```python
from build123d import *

# Parameters (mm, degrees)
SKETCH2_R           = 1
SKETCH2_R_2         = 7.975
BOSS_EXTRUDE1_DEPTH = 0.25


with BuildPart() as part:
    # Sketch2 → Boss-Extrude1 (new body)
    with BuildSketch(Plane.XY):
        with BuildLine():
            Line((-10.99049083, -10.599113396), (11.00950917, -10.599113396))
            ThreePointArc((11.00950917, -10.599113396), (12.70835196, -9.26915289), (11.825030389, -7.300751312))
            add(Edge.make_bspline(
                [(11.825030389, -7.300751312), (9.759593251, -6.043315053), (10.296923436, -3.493867271)],
                knots=[0, 0, 0, 1, 1, 1], degree=2))
            ThreePointArc((10.296923436, -3.493867271), (11.009509171, 0.400886603), (10.296923436, 4.295640477))
            add(Edge.make_bspline(
                [(10.296923436, 4.295640477), (9.75959325, 6.845088261), (11.825030389, 8.102524521)],
                knots=[0, 0, 0, 1, 1, 1], degree=2))
            ThreePointArc((11.825030389, 8.102524521), (12.70835196, 10.070926099), (11.00950917, 11.400886604))
            Line((11.00950917, 11.400886604), (-10.99049083, 11.400886604))
            ThreePointArc((-10.99049083, 11.400886604), (-12.689333619, 10.070926099), (-11.806012048, 8.102524521))
            add(Edge.make_bspline(
                [(-11.806012048, 8.102524521), (-9.740574911, 6.845088262), (-10.277905095, 4.29564048)],
                knots=[0, 0, 0, 1, 1, 1], degree=2))
            ThreePointArc((-10.277905095, 4.29564048), (-10.99049083, 0.400886606), (-10.277905095, -3.493867268))
            add(Edge.make_bspline(
                [(-10.277905095, -3.493867268), (-9.740574909, -6.043315053), (-11.806012048, -7.300751312)],
                knots=[0, 0, 0, 1, 1, 1], degree=2))
            ThreePointArc((-11.806012048, -7.300751312), (-12.689333619, -9.26915289), (-10.99049083, -10.599113396))
        make_face()
        with Locations((11.00950917, 9.650886604)):
            Circle(SKETCH2_R, mode=Mode.SUBTRACT)
        with Locations((-10.99049083, 9.650886604)):
            Circle(SKETCH2_R, mode=Mode.SUBTRACT)
        with Locations((11.00950917, -8.849113396)):
            Circle(SKETCH2_R, mode=Mode.SUBTRACT)
        with Locations((-10.99049083, -8.849113396)):
            Circle(SKETCH2_R, mode=Mode.SUBTRACT)
        with Locations((0.00950917, 0.400886604)):
            Circle(SKETCH2_R_2, mode=Mode.SUBTRACT)
    extrude(amount=BOSS_EXTRUDE1_DEPTH)


solid = part.part
```
Here's how the part is built. I have some questions about the finished solid (model axes, mm). Round coordinates to 2 decimals unless told otherwise and drop trailing zeros. Order: outer loops, then holes, each group sorted by start corner. A loop starts at its lowest first (then second) coordinate and runs counter-clockwise, first axis right, second up. Notation, with made-up numbers: (88.25, 11) -> (116.25, 11) arc R36 cw to (116.25, 48) -> close; hole circle Ø7 at (32, 6). An arc over 180 degrees is marked (long way). Use a Markdown table: item, result. Add a question column.
(1) I need wall thicknesses on line 1 along X through (y, z) = (0.5, 0.1); line 2 along X through (y, z) = (-9.5, 0.1); line 3 along X through (y, z) = (-9, 0.2). Which ranges of each line are inside material? Lowest first, please.
(2) Suppose I cut it at C-C, the plane z = 0.1. Count the separate pieces of the cut face and the enclosed holes in it, and give its area (3 significant figures).
(3) Suppose I cut it at A-A, the plane y = 0.75. Please give me the cut outline in (x, z), and give its area (3 significant figures).
(4) Suppose I cut it at B-B, the plane x = -4.25. Please give me the cut outline in (y, z), and give its area (3 significant figures).
Verdict:
| question | item | result |
|---|---|---|
| 1 | line 1 | -10.99 to -7.96, 7.98 to 11.01 |
| 1 | line 2 | -12.61 to -11.75, -10.23 to 10.25, 11.77 to 12.63 |
| 1 | line 3 | -12.73 to -11.98, -10 to 10.02, 12 to 12.75 |
| 2 | separate pieces | 1 |
| 2 | enclosed holes | 5 |
| 2 | area | 280 mm2 |
| 3 | outline | (-10.98, 0) -> (-7.96, 0) -> (-7.96, 0.25) -> (-10.98, 0.25) -> close; (7.98, 0) -> (11, 0) -> (11, 0.25) -> (7.98, 0.25) -> close |
| 3 | area | 1.51 mm2 |
| 4 | outline | (-10.6, 0) -> (-6.34, 0) -> (-6.34, 0.25) -> (-10.6, 0.25) -> close; (7.14, 0) -> (11.4, 0) -> (11.4, 0.25) -> (7.14, 0.25) -> close |
| 4 | area | 2.13 mm2 |
